Print and shaded views of the part. All mm, measured from the part's lowest x, y and z. Round coordinates to 2 decimals unless told otherwise and drop trailing zeros. Loops run counter-clockwise (first coordinate to the right, second up) from the corner with the lowest first, then second, coordinate; pieces in that order, holes last. Notation, with made-up numbers: (60, -22) -> (79, -22) arc R20 ccw to (79, 8) -> close; hole circle Ø9 at (6, -22.75). An arc over 180 degrees is marked (long way). Answer as CSV lines item,"result".
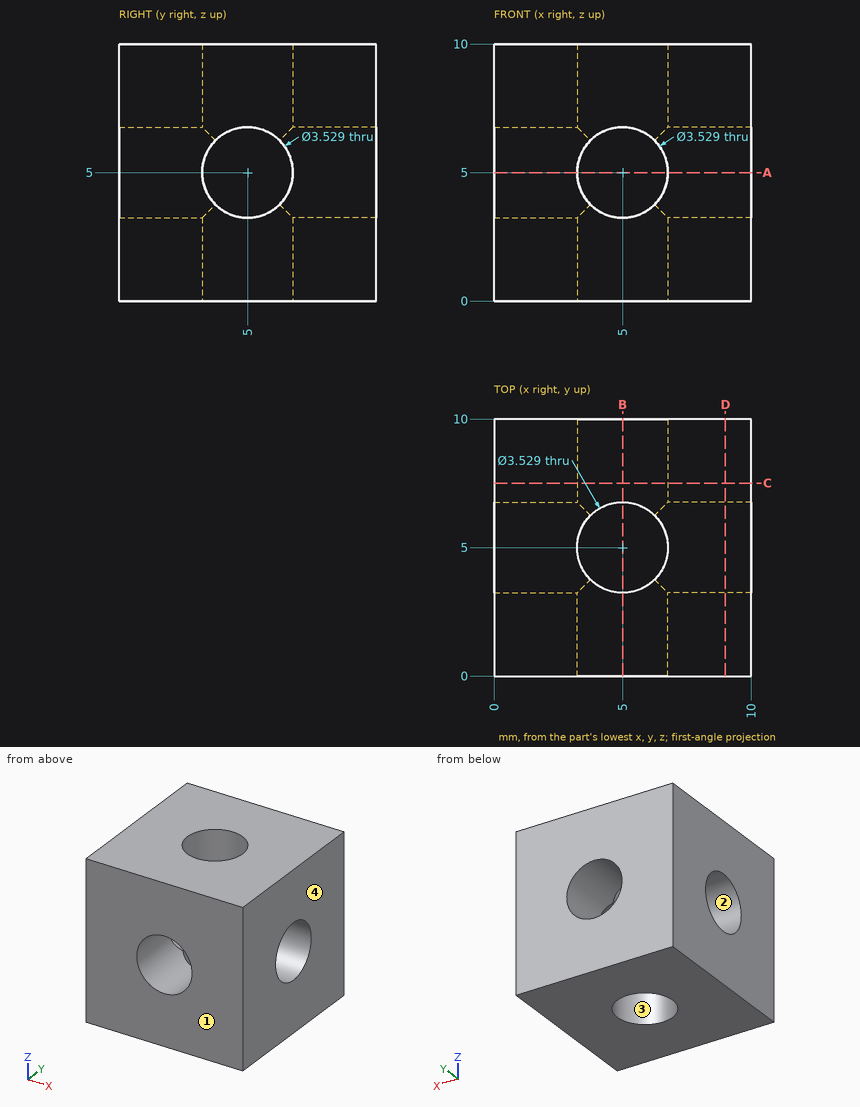
Q1. Drop flat-ended pins along their axis: pin 1 Ø5 at (x, y) = (8.5, 7) entering from -Z; pin 2 Ø2 at (x, y) = (5, 5) entering from -Z. Give the stop position or say it passes through.
Results:
pin 1,"z = 0"
pin 2,"through"
Q2. Two-plate mould, pull along Y, no slides. Class the marked faces 1, 2, 3 and 4: pulls with the +Y half, pulls with the -Y half, needs draft (parallel to the pull), parting line crosses it, or undercut.
Results:
face 1,"pulls with the -Y half"
face 2,"undercut"
face 3,"undercut"
face 4,"needs draft"
Q3. Slice it at C-C, the plane y = 7.5. Give the cut face in (x, z).
Results:
outline,"(0, 0) -> (10, 0) -> (10, 10) -> (0, 10) -> close; hole circle Ø3.53 at (5, 5)"
Q4. Probe L1, parallel to Z at x = 5, y = 7.35; L2, parallel to Y at x = 3.75, z = 3.5. List the from-to ranges inside material, lowest first. Write a range as [from, to].
Results:
L1,"[0, 3.24], [6.76, 10]"
L2,"[0, 3.75], [6.25, 10]"
Q5. Slice it at A-A, the plane z = 5. Give the cut face in (x, y), and give its area (3 significant figures).
Results:
outline,"(0, 0) -> (3.24, 0) -> (3.24, 3.24) -> (0, 3.24) -> close; (0, 6.76) -> (3.24, 6.76) -> (3.24, 10) -> (0, 10) -> close; (6.76, 0) -> (10, 0) -> (10, 3.24) -> (6.76, 3.24) -> close; (6.76, 6.76) -> (10, 6.76) -> (10, 10) -> (6.76, 10) -> close"
area,"41.9 mm2"
